Work out the finished part from the listing and answer in its coordinate system (mm). A direction names the side the tool comes from. Coordinates: 2 decimals unless noted, no trailing zeros. Order: outer loops, then holes, each group sorted by start corner. A loop starts at its lowest first (then second) coordinate and runs counter-clockwise, first axis right, second up.
1. The part is cut by section B-B, the plane x = -49. Give the vertices of the cut face in (y, z), then the cut area to 3 significant figures.
2. The part is cut by section C-C, the plane x = -34. Give the vertices of the cut face in (y, z).
3. Find the intervals of material crossed by probe 1 along Y at (x, z) = (-28, 64.5); probe 2 along Z at (x, y) = (-5.5, 12.5); probe 3 along Z at (x, y) = (-21.5, 11.25), in increasing order.
4. The part is cut by section D-D, the plane z = 70.5. Give the vertices of the cut face in (x, y).
5. Determine the mould class of faces 1 (the cylindrical face through (-6.35, 6.13, 32.89)), 2 (the flat face through (-55.88, 1, 45)), 3 (the flat face through (-28, -0.661, 53)) for opening direction X: +X half, -X half, draft (parallel to the pull), parting line (faces both ways), or undercut.
6. Flat-ended cylindrical pins translate along their axes: pin 1 Ø12 at (x, y) = (-32, 11.5) entering from -Z; pin 2 Ø1 at (x, y) = (-13, 18.5) entering from -Z; pin 3 Ø6 at (x, y) = (-43.5, 14) entering from -Z. Find the tip coordinate at first contact, or state that the pin passes through.
7. A tool of negligible diameter and unlimited length cuts with its end or side. For faces 4 (the cylindrical face through (-49.657, 22.27, 30.049)), 5 (the flat face through (-28, 1.839, 54)), from which of +Z, -Z, +X, -X, +Y, -Y can it reach the whole face along a straight path? Write none if from no direction.
8. The part is cut by section A-A, the plane z = 58.5. Give the vertices of the cut face in (x, y).
```python
from build123d import *

# Parameters (mm, degrees)
BOSS_EXTRUDE1_DEPTH = 55.88
SKETCH4_R           = 1.905
CUT_EXTRUDE1_DEPTH  = 42.418
SKETCH5_R           = 1.6256
CUT_EXTRUDE2_DEPTH  = 2.5


with BuildPart() as part:
    # Sketch3 → Boss-Extrude1 (new body)
    with BuildSketch(Plane(origin=(0, 0, 0), x_dir=(0, 0, -1), z_dir=(1, 0, 0))):
        Polygon((-72.719013739, -0.661158353), (-72.719013739, 1.838841647), (-34.938762817, 1.838841647), (-30.74863229, 25.602252727), (-28.286612908, 25.168132283), (-32.841013739, -0.661158353), align=None)
    extrude(amount=-BOSS_EXTRUDE1_DEPTH)

    # Sketch4 → Cut-Extrude1 (cut)
    with BuildSketch(Plane(origin=(0, 1.838841647, 0), x_dir=(1, 0, 0), z_dir=(0, 1, 0))):
        with Locations(Location((-40.386, -58.241013739, 0), (0, 0, 270))):
            Circle(SKETCH4_R)
        with Locations(Location((-15.494, -58.241013739, 0), (0, 0, 270))):
            Circle(SKETCH4_R)
    extrude(amount=-CUT_EXTRUDE1_DEPTH, mode=Mode.SUBTRACT)

    # Sketch5 → Cut-Extrude2 (cut)
    with BuildSketch(Plane(origin=(0, 5.596207749, 31.737671267), x_dir=(-1, 0, 0), z_dir=(0, -0.17364817766692642, -0.9848077530122088))):
        with Locations(Location((48.214905279, 15.963281142, 0), (0, 0, 90))):
            Circle(SKETCH5_R)
        with Locations(Location((7.7216, -0.546718858, 0), (0, 0, 90))):
            Circle(SKETCH5_R)
    extrude(amount=-CUT_EXTRUDE2_DEPTH, mode=Mode.SUBTRACT)


solid = part.part
```
Geometry says:
1. outline: (-0.66, 32.84) - (19.92, 29.21) - (20.35, 31.67) - (1.84, 34.94) - (1.84, 72.72) - (-0.66, 72.72) - close; (22.72, 28.72) - (25.17, 28.29) - (25.6, 30.75) - (23.15, 31.18) - close
1. area: 153 mm2
2. outline: (-0.66, 32.84) - (25.17, 28.29) - (25.6, 30.75) - (1.84, 34.94) - (1.84, 72.72) - (-0.66, 72.72) - close
3. probe 1: y = -0.66 to 1.84
3. probe 2: z = 30.52 to 33.06
3. probe 3: z = 30.74 to 33.28
4. outline: (-55.88, -0.66) - (0, -0.66) - (0, 1.84) - (-55.88, 1.84) - close
5. face 1: undercut
5. face 2: -X half
5. face 3: draft
6. pin 1: stops at z = 29.64
6. pin 2: stops at z = 29.37
6. pin 3: stops at z = 29.73
7. face 4: none
7. face 5: +Z, +X, -X, +Y
8. outline: (-55.88, -0.66) - (-42.27, -0.66) - (-42.27, 1.84) - (-55.88, 1.84) - close; (-38.5, -0.66) - (-17.38, -0.66) - (-17.38, 1.84) - (-38.5, 1.84) - close; (-13.61, -0.66) - (0, -0.66) - (0, 1.84) - (-13.61, 1.84) - close
